from build123d import *

# Parameters (mm, degrees)
SKETCH1_R           = 2
BOSS_EXTRUDE1_DEPTH = 5
SKETCH2_R           = 3
BOSS_EXTRUDE2_DEPTH = 8


with BuildPart() as part:
    # Sketch1 → Boss-Extrude1 (new body)
    with BuildSketch(Plane(origin=(0, 0, 0), x_dir=(1, 0, 0), z_dir=(0, 1, 0))):
        with BuildLine():
            Line((-34.19, -4), (34.19, -4))
            ThreePointArc((34.19, -4), (38.19, 0), (34.19, 4))
            Line((34.19, 4), (-34.19, 4))
            ThreePointArc((-34.19, 4), (-38.19, 0), (-34.19, -4))
        make_face()
        with Locations(Location((34.19, 0, 0), (0, 0, 270))):
            Circle(SKETCH1_R, mode=Mode.SUBTRACT)
        with Locations(Location((-34.19, 0, 0), (0, 0, 270))):
            Circle(SKETCH1_R, mode=Mode.SUBTRACT)
    extrude(amount=BOSS_EXTRUDE1_DEPTH)

    # Sketch2 → Boss-Extrude2 (add)
    with BuildSketch(Plane.XY.offset(4)):
        with BuildLine():
            ThreePointArc((-3.678488933, 13.386549744), (-12.35949887, 7.188806921), (-22.798898944, 5))
            Line((-22.798898944, 5), (6e-09, 5))
            Line((6e-09, 5), (22.798898944, 5))
            ThreePointArc((22.798898944, 5), (12.35949887, 7.188806921), (3.678488933, 13.386549744))
            ThreePointArc((3.678488933, 13.386549744), (0, 15), (-3.678488933, 13.386549744))
        make_face()
        with Locations((0, 10)):
            Circle(SKETCH2_R, mode=Mode.SUBTRACT)
    extrude(amount=-BOSS_EXTRUDE2_DEPTH)


solid = part.part
Geometry check sheet. Reference: the model listing, model coordinates, mm. A direction names the side the tool comes from. Give positions to 0.01 mm unless a question says otherwise; leave off trailing zeros. Order: outer loops, then holes, each group sorted by start corner. A loop starts at its lowest first (then second) coordinate and runs counter-clockwise, first axis right, second up. Notation, with made-up numbers: M -6,41.5 L 42,41.5 A16 ccw 42,61.5 Z; hole C -5,16 d4. An arc over 180 degrees is marked long. Use a Markdown table: item, result.
Item 1: Draft check along Z on faces 3 (the flat face through (-29, 5, 0)), 4 (the flat face through (0, 4, -4)), 5 (the cylindrical face through (32.416, 2.465, 0.923)). Enter one of: +Z half, -Z half, draft (parallel to the pull), parting line (faces both ways), or undercut.
Answers follow:
| item | result |
|---|---|
| face 3 | draft |
| face 4 | -Z half |
| face 5 | undercut |
Item 2: Section check B-B (y = 12.25). Record the cut outline in (x, z).
Answers follow:
| item | result |
|---|---|
| outline | M -4.79,-4 L -1.98,-4 L -1.98,4 L -4.79,4 Z; M 1.98,-4 L 4.79,-4 L 4.79,4 L 1.98,4 Z |
Item 3: Depth check by flat-ended pin: P1, Ø3, axis at x = 10.5, z = 2.5, coming from the -Y side. Enter the tip coordinate at first touch or a pass-through.
Answers follow:
| item | result |
|---|---|
| P1 | stops at y = 0 |
Item 4: Section check D-D (x = 23.5). Record the cut outline in (y, z), and give its area (3 significant figures).
Answers follow:
| item | result |
|---|---|
| outline | M 0,-4 L 5,-4 L 5,4 L 0,4 Z |
| area | 40.0 mm2 |
Item 5: Section check C-C (y = 2.5). Record the cut outline in (x, z), and give its area (3 significant figures).
Answers follow:
| item | result |
|---|---|
| outline | M -34.19,-4 L 34.19,-4 A4 ccw 34.19,4 L -34.19,4 A4 ccw Z; hole C -34.19,0 d4; hole C 34.19,0 d4 |
| area | 572 mm2 |
Item 6: Material ranges on line 1 along X through (y, z) = (3.25, 0); line 2 along Y through (x, z) = (0, 1.5); line 3 along Y through (x, z) = (32, -1), recorded low to high.
Answers follow:
| item | result |
|---|---|
| line 1 | x = -38.19 to -36.19, -32.19 to 32.19, 36.19 to 38.19 |
| line 2 | y = 0 to 7, 13 to 15 |
| line 3 | y = 0 to 5 |
Item 7: Tool access check on faces 1 (the flat face through (29, 5, 0)), 2 (the flat face through (-1, 0, 0)). Record the directions out of +Z, -Z, +X, -X, +Y, -Y that give a thin tool (end or side, any length) a straight path to the whole face; none if there is none.
Answers follow:
| item | result |
|---|---|
| face 1 | +Z, -Z, +X, +Y |
| face 2 | +Z, -Z, +X, -X, -Y |
Item 8: Section check A-A (z = 0). Record the cut outline in (x, y).
Answers follow:
| item | result |
|---|---|
| outline | M -38.19,0 L -36.19,0 L -36.19,5 L -38.19,5 Z; M -32.19,0 L 32.19,0 L 32.19,5 L 22.8,5 A25.99 cw 3.68,13.39 A5 ccw -3.68,13.39 A25.99 cw -22.8,5 L -32.19,5 Z; M 36.19,0 L 38.19,0 L 38.19,5 L 36.19,5 Z; hole C 0,10 d6 |
